Read the model definition and answer for the solid it produces. Units are mm, in the model's axes. A direction names the side the tool comes from. Round coordinates to 2 decimals unless told otherwise and drop trailing zeros. Return JSON: item names as keys, results as strings.
from build123d import *

# Parameters (mm, degrees)
SKETCH1_W                       = 105
SKETCH1_H                       = 85
SKETCH1_R                       = 4.2
BOSS_EXTRUDE1_DEPTH             = 10
SKETCH14_R                      = 18
SKETCH14_R_2                    = 17
BOSS_EXTRUDE4_DEPTH             = 700
BOSS_EXTRUDE4_DIRECTION_2_REACH = 70.283
RIB2_REACH                      = 716.562
SKETCH21_WALL_W                 = 1464.864259786
SKETCH21_WALL_H                 = 4
RIB5_REACH                      = 716.562
SKETCH22_WALL_W                 = 1457.169117376
SKETCH22_WALL_H                 = 4
FILLET1_R                       = 7
FILLET2_R                       = 7
CUT_EXTRUDE1_REACH              = 717.102
CUT_EXTRUDE1_END_RADIUS         = 17
SKETCH26_R                      = 4.1


with BuildPart() as part:
    # Sketch1 → Boss-Extrude1 (new body)
    with BuildSketch(Plane(origin=(0, 0, 0), x_dir=(1, 0, 0), z_dir=(0, 1, 0))):
        Rectangle(SKETCH1_W, SKETCH1_H)
        with Locations(Location((-40, -30, 0), (0, 0, 270))):
            Circle(SKETCH1_R, mode=Mode.SUBTRACT)
        with Locations(Location((40, 30, 0), (0, 0, 270))):
            Circle(SKETCH1_R, mode=Mode.SUBTRACT)
        with Locations(Location((40, -30, 0), (0, 0, 270))):
            Circle(SKETCH1_R, mode=Mode.SUBTRACT)
        with Locations(Location((-40, 30, 0), (0, 0, 270))):
            Circle(SKETCH1_R, mode=Mode.SUBTRACT)
    extrude(amount=BOSS_EXTRUDE1_DEPTH)

    # Sketch14 → Boss-Extrude4 (add)
    with BuildSketch(Plane(origin=(0, 10, 0), x_dir=(-0.9961946980917459, -0.08715574274765506, 0), z_dir=(0.08715574274765506, -0.9961946980917459, 0))):
        with Locations((0.435778714, 0)):
            Circle(SKETCH14_R)
        with Locations((0.435778714, 0)):
            Circle(SKETCH14_R_2, mode=Mode.SUBTRACT)
    extrude(amount=-BOSS_EXTRUDE4_DEPTH)

    # Boss-Extrude4 direction 2: up to this face of the body (flat: up to its plane)
    boss_extrude4_direction_2_end = Plane(part.part.faces().sort_by_distance((0, 10, 0))[0])
    # Sketch14 → Boss-Extrude4 direction 2 (add, up to the picked face)
    with BuildSketch(Plane(origin=(0, 10, 0), x_dir=(-0.9961946980917459, -0.08715574274765506, 0), z_dir=(0.08715574274765506, -0.9961946980917459, 0)), mode=Mode.PRIVATE) as boss_extrude4_direction_2_sk1:
        with Locations((0.435778714, 0)):
            Circle(SKETCH14_R)
        with Locations((0.435778714, 0)):
            Circle(SKETCH14_R_2, mode=Mode.SUBTRACT)
    boss_extrude4_direction_2_tool1 = split(extrude(boss_extrude4_direction_2_sk1.sketch, amount=BOSS_EXTRUDE4_DIRECTION_2_REACH, mode=Mode.PRIVATE), bisect_by=boss_extrude4_direction_2_end, keep=Keep.BOTH, mode=Mode.PRIVATE)
    add(boss_extrude4_direction_2_tool1.solids().sort_by(Axis((16.990205, 11.48645, 0), (0.08715574274765506, -0.9961946980917459, 0)))[0])

    # Sketch21 wall → Rib2 (add, up to next)
    with BuildSketch(Plane(origin=(27.942090865, 21.517823641, 0), x_dir=(0.730658017889, -0.682743627502, 0), z_dir=(0.682743627502, 0.730658017889, 0)), mode=Mode.PRIVATE) as rib2_sk1:
        Rectangle(SKETCH21_WALL_W, SKETCH21_WALL_H)
    rib2_tool1 = extrude(rib2_sk1.sketch, amount=-RIB2_REACH, mode=Mode.PRIVATE) - part.part
    add(rib2_tool1.solids().sort_by_distance((27.942090865, 21.517823641, 0))[0])

    # Sketch22 wall → Rib5 (add, up to next)
    with BuildSketch(Plane(origin=(-28.227154914, 20.343956887, 0), x_dir=(-0.607494293968, -0.794324041432, 0), z_dir=(0.794324041432, -0.607494293968, 0)), mode=Mode.PRIVATE) as rib5_sk1:
        Rectangle(SKETCH22_WALL_W, SKETCH22_WALL_H)
    rib5_tool1 = extrude(rib5_sk1.sketch, amount=RIB5_REACH, mode=Mode.PRIVATE) - part.part
    add(rib5_tool1.solids().sort_by_distance((-28.227154914, 20.343956887, 0))[0])

    # Fillet1
    fillet1_edges = [part.edges().sort_by_distance(p)[0] for p in [
        (52.5, 10, 0),
        (-52.5, 10, 0),
        (52.5, 5, 42.5),
        (-52.5, 5, 42.5),
    ]]
    fillet(fillet1_edges, radius=FILLET1_R)

    # Fillet2
    # the kernel refuses this fillet: 7 mm, written as the material it takes off along each edge
    with BuildSketch(Plane(origin=(45.5, 3, 35.5), x_dir=(0, 1, 0), z_dir=(0, 0, 1))) as fillet2_piece_1_section:
        Polygon((0, 0), (FILLET2_R, 0), (FILLET2_R, -FILLET2_R), (0, -FILLET2_R), align=None)
    fillet2_piece_1 = extrude(amount=FILLET2_R, mode=Mode.PRIVATE)
    fillet2_piece_1 = fillet2_piece_1 - Plane(origin=(45.5, 3, 35.5), x_dir=(-0.7071067811865475, -0.7071067811865475, 0), z_dir=(0, 0, 1)) * Sphere(FILLET2_R, mode=Mode.PRIVATE)
    add(fillet2_piece_1, mode=Mode.SUBTRACT)
    with BuildSketch(Plane(origin=(-45.5, 3, 35.5), x_dir=(0, 1, 0), z_dir=(0, 0, 1))) as fillet2_piece_2_section:
        Polygon((0, 0), (FILLET2_R, 0), (FILLET2_R, FILLET2_R), (0, FILLET2_R), align=None)
    fillet2_piece_2 = extrude(amount=FILLET2_R, mode=Mode.PRIVATE)
    fillet2_piece_2 = fillet2_piece_2 - Plane(origin=(-45.5, 3, 35.5), x_dir=(0.7071067811865475, -0.7071067811865475, 0), z_dir=(0, 0, 1)) * Sphere(FILLET2_R, mode=Mode.PRIVATE)
    add(fillet2_piece_2, mode=Mode.SUBTRACT)
    with BuildSketch(Plane(origin=(-45.5, 10, -42.5), x_dir=(0, 0, 1), z_dir=(1, 0, 0))) as fillet2_piece_3:
        with BuildLine():
            CenterArc((FILLET2_R, FILLET2_R), FILLET2_R, 180, 90)
            Line((0, FILLET2_R), (0, 0))
            Line((0, 0), (FILLET2_R, 0))
        make_face()
    extrude(amount=91, mode=Mode.SUBTRACT)
    with BuildSketch(Plane(origin=(45.5, 10, 42.5), x_dir=(0, -1, 0), z_dir=(-1, 0, 0))) as fillet2_piece_4:
        with BuildLine():
            CenterArc((FILLET2_R, -FILLET2_R), FILLET2_R, 90, 90)
            Line((0, -FILLET2_R), (0, 0))
            Line((0, 0), (FILLET2_R, 0))
        make_face()
    extrude(amount=91, mode=Mode.SUBTRACT)
    with BuildSketch(Plane(origin=(-52.5, -17.5, -42.5), x_dir=(0, 0, 1), z_dir=(0, 1, 0))) as fillet2_piece_5:
        with BuildLine():
            CenterArc((FILLET2_R, FILLET2_R), FILLET2_R, 180, 90)
            Line((0, FILLET2_R), (0, 0))
            Line((0, 0), (FILLET2_R, 0))
        make_face()
    extrude(amount=20.5, mode=Mode.SUBTRACT)
    with BuildSketch(Plane(origin=(52.5, -17.5, -42.5), x_dir=(0, 0, 1), z_dir=(0, 1, 0))) as fillet2_piece_6:
        with BuildLine():
            CenterArc((FILLET2_R, -FILLET2_R), FILLET2_R, 90, 90)
            Line((0, -FILLET2_R), (0, 0))
            Line((0, 0), (FILLET2_R, 0))
        make_face()
    extrude(amount=20.5, mode=Mode.SUBTRACT)
    with BuildSketch(Plane(origin=(-45.5, 3, -42.5), x_dir=(-1, 0, 0), z_dir=(0, -1, 0))) as fillet2_piece_7:
        with BuildLine():
            CenterArc((7 - FILLET2_R, -FILLET2_R), FILLET2_R, 0, 90)
            Line((7, -FILLET2_R), (7, 0))
            Line((7, 0), (7 - FILLET2_R, 0))
        make_face()
    revolve(axis=Axis((-45.5, 3, -42.5), (0, 0, -1)), revolution_arc=90, mode=Mode.SUBTRACT)
    with BuildSketch(Plane(origin=(45.5, 3, -42.5), x_dir=(1, 0, 0), z_dir=(0, -1, 0))) as fillet2_piece_8:
        with BuildLine():
            CenterArc((7 - FILLET2_R, FILLET2_R), FILLET2_R, 270, 90)
            Line((7, FILLET2_R), (7, 0))
            Line((7, 0), (7 - FILLET2_R, 0))
        make_face()
    revolve(axis=Axis((45.5, 3, -42.5), (0, 0, 1)), revolution_arc=90, mode=Mode.SUBTRACT)

    # Cut-Extrude1: up to this cylinder (the profile starts outside it)
    cut_extrude1_end = Plane(origin=(-57.085353251, 657.488573385, 0), z_dir=(-0.08715574274765504, 0.9961946980917459, 0)) * Cylinder(CUT_EXTRUDE1_END_RADIUS, 1469.204, mode=Mode.PRIVATE)
    # Sketch26 → Cut-Extrude1 (cut, up to the surface)
    with BuildSketch(Plane(origin=(-17.497384121, -1.530822752, 0), x_dir=(0, 0, 1), z_dir=(-0.9961946980917459, -0.08715574274765504, 0)), mode=Mode.PRIVATE) as cut_extrude1_sk1:
        with Locations(Location((0, 659.961946981, 0), (0, 0, 270))):
            Circle(SKETCH26_R)
    cut_extrude1_tool1 = extrude(cut_extrude1_sk1.sketch, amount=-CUT_EXTRUDE1_REACH, mode=Mode.PRIVATE) - cut_extrude1_end
    add(cut_extrude1_tool1.solids().sort_by_distance((-75.016858, 655.91977, 0))[0], mode=Mode.SUBTRACT)


solid = part.part
Item 1: For a pull along Z with two mould halves and no side action, classify faces 1 (the cylindrical face through (-47.864, 361.312, 6.894)), 2 (the flat face through (27.708, 21.737, -0.028)), 3 (the cylindrical face through (-46.09, 351.65, 6.51)), 4 (the flat face through (-1, 10, 0)) as released by +Z, released by -Z, zero draft, split by the parting line, or undercut.
Worked answers:
{"face 1": "split by the parting line", "face 2": "zero draft", "face 3": "undercut", "face 4": "undercut"}
Item 2: Straight lines are drawn through the part: L1, parallel to X at y = 3.5, z = 30; L2, parallel to X at y = 7, z = -30; L3, parallel to Y at x = 12.5, z = -35. For each, find the intervals that lie inside material, in ascending order. Write a range as [from, to].
Worked answers:
{"L1": "x = [-52.48, -44.2], [-35.8, 35.8], [44.2, 52.48]", "L2": "x = [-51.24, -44.2], [-35.8, 35.8], [44.2, 51.24]", "L3": "y = [0, 10]"}
Item 3: Flat-ended cylindrical pins translate along their axes: pin 1 (10 mm diameter, centred on x = -43, y = 341.5, fed in from +Z); pin 2 (18.5 mm diameter, centred on x = 28.5, y = 26, fed in from +Z); pin 3 (5.5 mm diameter, centred on x = -30.5, y = 21, fed in from -Z). Find the tip coordinate at first contact, or state that the pin passes through.
Worked answers:
{"pin 1": "stops at z = 15.86", "pin 2": "stops at z = 2", "pin 3": "stops at z = -2"}
Item 4: A tool of negligible diameter and unlimited length cuts with its end or side. For faces 5 (the flat face through (-11, 10, 15)), 6 (the flat face through (-24, 17, -2)), 7 (the flat face through (24, 17, 2)), from which of +Z, -Z, +X, -X, +Y, -Y can it reach the whole face along a straight path? Write none if from no direction.
Worked answers:
{"face 5": "none", "face 6": "-Z, -X", "face 7": "+Z, +X, +Y"}
